from build123d import *

# Parameters (mm, degrees)
F0_W     = 7.9375
F0_H     = 6.35
F1_DEPTH = 9.525
F3_W     = 7.9375
F3_H     = 10.31875
F4_DEPTH = 3.175
F5_R     = 2.778125
F6_DEPTH = 11.43


with BuildPart() as f1:
    # F0 (on Front) → F1 (new body)
    with BuildSketch(Plane.XZ):
        with Locations((-15.998094, -4.638754)):
            Rectangle(F0_W, F0_H)
        with BuildLine():
            ThreePointArc((-15.998094, 2.504996), (-18.804425, 1.342576), (-19.966844, -1.463754))
            Line((-19.966844, -1.463754), (-12.029344, -1.463754))
            ThreePointArc((-12.029344, -1.463754), (-13.191764, 1.342576), (-15.998094, 2.504996))
        make_face()
    extrude(amount=F1_DEPTH)

    # F3 (on face) → F4 (join)
    with BuildSketch(Plane.XZ.offset(9.525)):
        with Locations((-15.998094, -2.654379)):
            Rectangle(F3_W, F3_H)
    extrude(amount=F4_DEPTH)

    # F5 (on face) → F6 (cut)
    with BuildSketch(Plane.XZ.offset(12.7)):
        with Locations((-15.998094, -1.066879)):
            Circle(F5_R)
    extrude(amount=-F6_DEPTH, mode=Mode.SUBTRACT)


solid = f1.part
Source: CAD feature listing. Evaluate the final solid. Frame: model axes, mm. A direction names the side the tool comes from. Coordinates: 2 decimals unless noted, no trailing zeros. Order: outer loops, then holes, each group sorted by start corner. A loop starts at its lowest first (then second) coordinate and runs counter-clockwise, first axis right, second up. Notation, with made-up numbers: M -33,-25 L 21,-25 A20 cw 21,-21 Z; hole C -16,82.25 d7. An arc over 180 degrees is marked long. Write each question's results on one line, items separated by ' | '. Start each with the question number.
1. Section B-B, the plane z = -3.25. Return the cut outline in (x, y).
2. Section C-C, the plane x = -15.5. Return the cut outline in (y, z) (3 decimals), then the cut area to 3 significant figures.
3. Material intervals for L1, parallel to Y at x = -19.5, z = 0.75 (3 decimals); L2, parallel to X at y = -10, z = -3.25; L3, parallel to Z at x = -17.25, y = -10.5 (3 decimals), sorted ascending.
4. Section A-A, the plane y = -8.5. Return the cut outline in (x, z) (1 decimal).
5. Section D-D, the plane z = 1.25. Return the cut outline in (x, y) (3 decimals), then the cut area to 3 significant figures.
6. Pin query (flat end, axial travel): pin 1 (3 mm diameter, centred on x = -16, z = 0, fed in from -Y); pin 2 (3 mm diameter, centred on x = -18.5, y = -7.5, fed in from +Z). Return the tip coordinate at first contact, or that it passes through.
7. Reachability of faces 1 (the face through (-16, -1.27, -1)), 2 (the face through (-19, -9.525, 2)), 3 (the face through (-13, -9.525, 2)) from +Z, -Z, +X, -X, +Y, -Y: full face, straight path, thin tool, end or side. Return the list, or none.
8. Draft query along X for faces 4 (the face through (-19.967, -6, -4)), 5 (the face through (-13.35, -7.07, -0.23)), 6 (the face through (-16, 0, -3)). Return one class per face: +X half, -X half, draft (parallel to the pull), parting line (faces both ways), or undercut.
Solution:
1) outline: M -19.97,-12.7 L -17.72,-12.7 L -17.72,-1.27 L -14.28,-1.27 L -14.28,-12.7 L -12.03,-12.7 L -12.03,0 L -19.97,0 Z
2) outline: M -12.7,-7.814 L 0,-7.814 L 0,2.474 L -9.525,2.474 L -9.525,2.505 L -12.7,2.505 L -12.7,1.666 L -1.27,1.666 L -1.27,-3.8 L -12.7,-3.8 Z | area: 68.3 mm²
3) L1: -12.7 to -9.525 | L2: -19.97 to -17.72, -14.28 to -12.03 | L3: -7.814 to -3.547, 1.413 to 2.505
4) outline: M -20,-7.8 L -12,-7.8 L -12,-1.5 A4 ccw -16,2.5 A4 ccw -20,-1.5 Z; hole C -16,-1.1 d5.6
5) outline: M -19.967,-12.7 L -17.531,-12.7 L -17.531,-1.27 L -14.465,-1.27 L -14.465,-12.7 L -12.029,-12.7 L -12.029,-9.525 L -13.102,-9.525 L -13.102,0 L -18.894,0 L -18.894,-9.525 L -19.967,-9.525 Z | area: 45.3 mm²
6) pin 1: y = -1.27 | pin 2: z = 2.38
7) face 1: -Y | face 2: +Z, -X, +Y | face 3: +Z, +X, +Y
8) face 4: -X half | face 5: undercut | face 6: draft
